The listing builds one solid part. Answer for the finished solid, in the listing's coordinates (mm). A direction names the side the tool comes from. Give positions to 0.01 mm unless a question says otherwise; leave off trailing zeros. Loops run counter-clockwise (first coordinate to the right, second up) from the corner with the lowest first, then second, coordinate; pieces in that order, holes last. Notation, with made-up numbers: (-7, -29.5) - (8, -29.5) arc R25 ccw to (8, 1.5) - close; hole circle Ø7 at (-18.5, 59.5). An arc over 180 degrees is marked (long way). One line per item, written item: value. Start each with the question number.
from build123d import *

# Parameters (mm, degrees)
EXTRUDE003_DEPTH = 20
EXTRUDE002_DEPTH = 20
FILLET_R         = 2


with BuildPart() as extrude003:
    # Sketch004 (on Extrude) → Extrude003 (new body, symmetric)
    with BuildSketch(Plane.YZ):
        Polygon((20, 0), (-20, 0), (-20, 64), (-22, 66), (-22, 70), (-16, 64), (-16, 4), (16, 4), (16, 64), (22, 70), (22, 66), (20, 64), align=None)
    extrude(amount=EXTRUDE003_DEPTH, both=True)


with BuildPart() as bin:
    # Sketch003 → Extrude002 (new body, symmetric)
    with BuildSketch(Plane.XZ):
        Polygon((-20, 0), (20, 0), (20, 64), (22, 66), (22, 70), (16, 64), (16, 4), (-16, 4), (-16, 64), (-22, 70), (-22, 66), (-20, 64), align=None)
    extrude(amount=EXTRUDE002_DEPTH, both=True)

    # Fusion001: union Extrude003
    add(extrude003.part)

    # Fillet
    fillet_edges = [bin.edges().sort_by_distance(p)[0] for p in [
        (-20, 0, 0),
        (-16, 0, 64),
        (0, 20, 0),
        (20, 0, 0),
        (0, -20, 0),
        (0, 16, 64),
        (-16, 0, 4),
        (0, -16, 64),
        (0, 16, 4),
        (16, 0, 64),
        (0, -16, 4),
        (16, 0, 4),
    ]]
    fillet(fillet_edges, radius=FILLET_R)


solid = bin.part
1. Find the intervals of material crossed by L1, parallel to X at y = 9.5, z = 60.5; L2, parallel to Z at x = 12, y = 13.5, in increasing order. Write a range as [from, to].
2. A cutting plane is placed at A-A (z = 19). Determine the outline of the cut face in (x, y), plus the area to 3 significant figures.
3. Determine the mould class of faces 3 (the cylindrical face through (19.4, -0.28, 0.57)), 4 (the flat face through (0, -21, 65)), 5 (the cylindrical face through (-0.22, -15.4, 4.57)), 6 (the flat face through (0, 22, 68)) for opening direction Y: released by +Y, released by -Y, zero draft, split by the parting line, or undercut.
4. For faces 1 (the cylindrical face through (-0.23, -16.15, 63.93)), 2 (the flat face through (22, 0, 68)), determine the directions among +Z, -Z, +X, -X, +Y, -Y from which every point of the face is accessible in a straight line to the end or side of a thin tool.
5. A cutting plane is placed at B-B (x = 10). Determine the outline of the cut face in (y, z), plus the area to 3 significant figures.
6. Flat-ended cylindrical pins translate along their axes: pin 1 (2 mm diameter, centred on y = -15.5, z = 56, fed in from -X); pin 2 (9.5 mm diameter, centred on y = 5.5, z = 41, fed in from +X); pin 3 (0.6 mm diameter, centred on x = 20.5, z = 65.5, fed in from -Y). Find the tip coordinate at first contact, or state that the pin passes through.
7. A cutting plane is placed at D-D (x = -19). Determine the outline of the cut face in (y, z), plus the area to 3 significant figures.
Results below:
1. L1: x = [-20, -16], [16, 20]
1. L2: z = [0, 4]
2. outline: (-20, -20) - (20, -20) - (20, 20) - (-20, 20) - close; hole (-16, -16) - (16, -16) - (16, 16) - (-16, 16) - close
2. area: 576 mm^2
3. face 3: zero draft
3. face 4: released by -Y
3. face 5: undercut
3. face 6: released by +Y
4. face 1: +Z
4. face 2: +Z, -Z, +X, +Y, -Y
5. outline: (-22, 66) - (-20, 64) - (-20, 2) arc R2 ccw to (-18, 0) - (18, 0) arc R2 ccw to (20, 2) - (20, 64) - (22, 66) - (22, 70) - (16.59, 64.59) arc R2 ccw to (16, 63.17) - (16, 6) arc R2 cw to (14, 4) - (-14, 4) arc R2 cw to (-16, 6) - (-16, 63.17) arc R2 ccw to (-16.59, 64.59) - (-22, 70) - close
5. area: 672 mm^2
6. pin 1: stops at x = -20
6. pin 2: stops at x = 20
6. pin 3: stops at y = -20
7. outline: (-22, 66) - (-20, 64) - (-20, 2) arc R2 ccw to (-19, 0.27) - (19, 0.27) arc R2 ccw to (20, 2) - (20, 64) - (22, 66) - (22, 70) - (19, 67) - (-19, 67) - (-22, 70) - close
7. area: 2,690 mm^2
